Part model, mm, in its own coordinate system. A direction names the side the tool comes from. Give positions to 0.01 mm unless a question says otherwise; leave off trailing zeros. Write each loop counter-clockwise with the first axis right and the second up, starting at its lowest first coordinate (ties: lowest second). Pieces come first, ordered by that corner, then holes. Notation, with made-up numbers: (-27, -32.5) - (17, -32.5) arc R11 cw to (17, -26.5) - close; hole circle Ø8 at (-27.75, 46). An arc over 180 degrees is marked (long way). Answer as a JSON object with one key per item and string values. Group by question number.
```python
from build123d import *

# Parameters (mm, degrees)
SKETCH3_W           = 6.096
SKETCH3_H           = 6.096
BOSS_EXTRUDE1_DEPTH = 5.715
SKETCH4_R           = 1.7145
BOSS_EXTRUDE2_DEPTH = 1.3208
SKETCH5_W           = 12.7
SKETCH5_H           = 12.7
BOSS_EXTRUDE4_DEPTH = 2.667


with BuildPart() as part:
    # Sketch3 → Boss-Extrude1 (new, symmetric)
    with BuildSketch(Plane.XY):
        Rectangle(SKETCH3_W, SKETCH3_H)
    extrude(amount=BOSS_EXTRUDE1_DEPTH, both=True)

    # Sketch4 → Boss-Extrude2 (add)
    with BuildSketch(Plane.XY.offset(5.715)):
        Circle(SKETCH4_R)
    boss_extrude2 = extrude(amount=BOSS_EXTRUDE2_DEPTH)

    # Mirror1: Boss-Extrude2 across plane
    add(boss_extrude2.mirror(Plane.XY))

    # Sketch5 → Boss-Extrude4 (add, symmetric)
    with BuildSketch(Plane.XY):
        Rectangle(SKETCH5_W, SKETCH5_H)
    extrude(amount=BOSS_EXTRUDE4_DEPTH, both=True)


solid = part.part
```
1) Band-saw the part on C-C (z = 6.25). List the corners of the cut face in (x, y), plus the area to 3 significant figures.
2) Band-saw the part on D-D (x = -2.5). List the corners of the cut face in (y, z) (3 decimals).
3) Drop flat-ended pins along their axis: P1, Ø3, axis at y = 0.5, z = 5.5, coming from the -X side; P2, Ø2, axis at x = -4.5, y = 3.5, coming from the +Z side; P3, Ø1.5, axis at x = -1.5, z = 4, coming from the -Y side. Give the stop position or say it passes through.
4) Which spindle directions (+Z, -Z, +X, -X, +Y, -Y) get a long thin tool onto all of the face, cutting with end or side? Do faces 1 (the cylindrical face through (-0.372, -1.674, -6.366)), 2 (the flat face through (-3.048, 0, 4)), 3 (the flat face through (0, 3.048, 4)). Say none if no direction does.
5) Probe line 1 (Z direction, x = -1.75, y = 4); line 2 (X direction, y = -0.5, z = -5.5); line 3 (Z direction, x = 2.5, y = -2.25) (3 decimals). List the from-to ranges inside material, lowest first.
Verdict:
{
 "1": {"outline": "circle Ø3.43 at (0, 0)", "area": "9.23 mm2"},
 "2": {"outline": "(-6.35, -2.667) - (-3.048, -2.667) - (-3.048, -5.715) - (3.048, -5.715) - (3.048, -2.667) - (6.35, -2.667) - (6.35, 2.667) - (3.048, 2.667) - (3.048, 5.715) - (-3.048, 5.715) - (-3.048, 2.667) - (-6.35, 2.667) - close"},
 "3": {"P1": "x = -3.05", "P2": "z = 2.67", "P3": "y = -3.05"},
 "4": {"face 1": "-Z", "face 2": "+Z, -X, +Y, -Y", "face 3": "+Z, +X, -X, +Y"},
 "5": {"line 1": "-2.67 to 2.67", "line 2": "-3.05 to 3.05", "line 3": "-5.715 to 5.715"}
}
